Study the drawing (mm; zero at the part's minimum x, y, z) and answer. A direction names the side the tool comes from. Give positions to 0.01 mm unless a question says otherwise; leave off trailing zeros. Write each loop counter-clockwise with the first axis right and the second up, starting at its lowest first coordinate (ties: lowest second). Pieces come first, ordered by that corner, then holes. Notation, with made-up numbers: (20, 42) - (49, 42) arc R34 ccw to (49, 74) - close; hole circle Ø6 at (26.25, -28.75). An arc over 180 degrees is marked (long way). Answer in a Markdown table with one row per item. Add a question column.
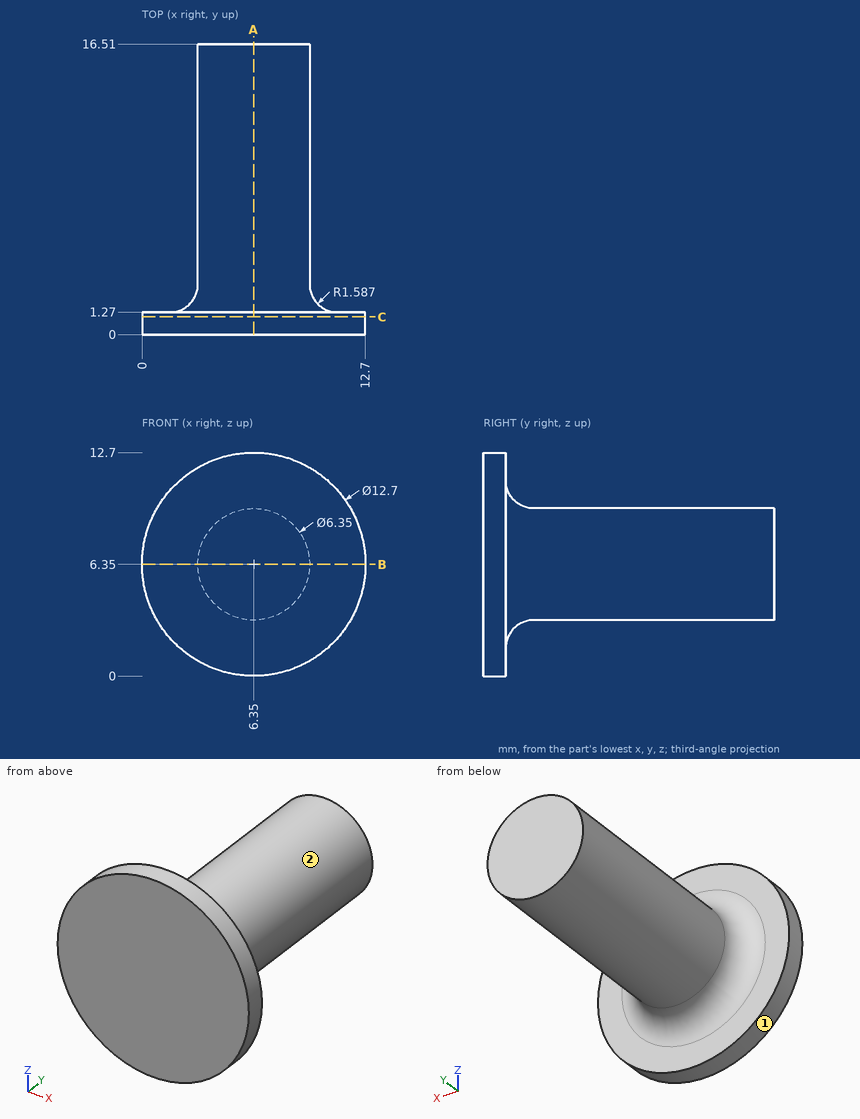
1. Section C-C (y = 1) is taken. Give the vertices of the cut face in (x, z), and give its area (3 significant figures).
2. Section A-A (x = 6.35) is taken. Give the vertices of the cut face in (y, z) (1 decimal), and give its area (3 significant figures).
3. A tool of negligible diameter and unlimited length cuts with its end or side. For the marked faces 1 and 2, from which of +Z, -Z, +X, -X, +Y, -Y can it reach the whole face along a straight path? Write none if from no direction.
4. Section B-B (z = 6.35) is taken. Give the vertices of the cut face in (x, y) (1 decimal), and give its area (3 significant figures).
5. Straight lines are drawn through the part: L1, parallel to Y at x = 11, z = 6.75; L2, parallel to X at y = 10.25, z = 6.5; L3, parallel to Z at x = 4.5, y = 5.5. For each, find the intervals that lie inside material, in ascending order. Write a range as [from, to].
6. Given pin 1 Ø1 at (x, z) = (4, 9.5) entering from +Y (1 decimal); pin 2 Ø4 at (x, z) = (6.5, 3) entering from +Y; pin 3 Ø6 at (y, z) = (12, 8) entering from +X (1 decimal); pin 4 Ø1.5 at (x, z) = (4, 11) entering from +Y, each flat-ended and moving along its own axis, determine where each tip first touches the part or whether it passes through.
Geometry check:
| question | item | result |
|---|---|---|
| 1 | outline | circle Ø12.7 at (6.35, 6.35) |
| 1 | area | 127 mm² |
| 2 | outline | (0, 0) - (1.3, 0) - (1.3, 1.6) arc R1.6 cw to (2.9, 3.2) - (16.5, 3.2) - (16.5, 9.5) - (2.9, 9.5) arc R1.6 cw to (1.3, 11.1) - (1.3, 12.7) - (0, 12.7) - close |
| 2 | area | 114 mm² |
| 3 | face 1 | +Y, -Y |
| 3 | face 2 | +Y |
| 4 | outline | (0, 0) - (12.7, 0) - (12.7, 1.3) - (11.1, 1.3) arc R1.6 cw to (9.5, 2.9) - (9.5, 16.5) - (3.2, 16.5) - (3.2, 2.9) arc R1.6 cw to (1.6, 1.3) - (0, 1.3) - close |
| 4 | area | 114 mm² |
| 5 | L1 | [0, 1.27] |
| 5 | L2 | [3.18, 9.52] |
| 5 | L3 | [3.77, 8.93] |
| 6 | pin 1 | y = 2 |
| 6 | pin 2 | y = 16.51 |
| 6 | pin 3 | x = 9.5 |
| 6 | pin 4 | y = 1.3 |
